Can you work these out from the model? Positions are in its coordinate system, mm. A direction names the side the tool comes from. Round coordinates to 2 decimals unless told otherwise and drop trailing zeros. Loops run counter-clockwise (first coordinate to the right, second up) from the corner with the lowest first, then second, coordinate; pieces in that order, holes last. Notation, with made-up numbers: M 41,-31.5 L 79,-31.5 A7 ccw 79,-23.5 Z; hole C -9.5,-21.5 d8. An arc over 180 degrees is marked long. Return JSON: item names as keys, results as strings.
```python
from build123d import *

# Parameters (mm, degrees)
SKETCH004_R           = 13
SKETCH004_R_2         = 1.6
PAD001_DEPTH          = 3
POLARPATTERN001_COUNT = 3
SKETCH005_R           = 16
SKETCH005_R_2         = 13
PAD002_DEPTH          = 3
CHAMFER003_SIZE       = 0.75


with BuildPart() as part:
    # Sketch004 (on Face1 of Binder001) → Pad001 (new body)
    with BuildSketch(Plane.XZ.offset(-1.75)):
        with BuildLine():
            ThreePointArc((19.050853, 6.088102), (-19.94876, -1.430732), (19.724681, -3.307108))
            Line((24.422075, -4.094689), (19.724681, -3.307108))
            ThreePointArc((24.422075, -4.094689), (31.398835, 2.251935), (23.587776, 7.537972))
            Line((23.587776, 7.537972), (19.050853, 6.088102))
        make_face()
        Circle(SKETCH004_R, mode=Mode.SUBTRACT)
        with Locations((25.414207, 1.822716)):
            Circle(SKETCH004_R_2, mode=Mode.SUBTRACT)
    pad001 = extrude(amount=PAD001_DEPTH)

    # PolarPattern001: Pad001 ×3 about axis
    polarpattern001_axis = Axis((0, 1.75, 0), (0, -1, 0))
    for i in range(1, POLARPATTERN001_COUNT):
        add(pad001.rotate(polarpattern001_axis, i * 360 / POLARPATTERN001_COUNT))

    # Sketch005 (on Face17 of PolarPattern001) → Pad002 (join)
    with BuildSketch(Plane.XZ.offset(1.25)):
        Circle(SKETCH005_R)
        Circle(SKETCH005_R_2, mode=Mode.SUBTRACT)
    extrude(amount=PAD002_DEPTH)

    # Chamfer003
    chamfer003_edges = [part.edges().sort_by_distance(p)[0] for p in [
        (-16, -4.25, 0),
        (31.398835, 1.75, 2.251935),
        (22.073378, 1.75, -3.700898),
        (11.21343, 1.75, -16.560767),
        (-4.759394, 1.75, -21.869587),
        (-13.749184, 1.75, -28.318156),
        (-14.241761, 1.75, -17.265657),
        (-19.94876, 1.75, -1.430732),
        (-16.55992, 1.75, 15.05655),
        (-17.64965, 1.75, 26.066221),
        (-7.831617, 1.75, 20.966555),
        (8.73533, 1.75, 17.991498),
        (21.319315, 1.75, 6.813037),
        (6.5, 1.75, 11.25833),
        (-13, 1.75, 0),
        (6.5, 1.75, -11.25833),
        (23.814207, 1.75, 1.822716),
        (-13.485622, 1.75, 19.71235),
        (-10.328585, 1.75, -21.535066),
    ]]
    chamfer(chamfer003_edges, length=CHAMFER003_SIZE)


solid = part.part
```
Q1. On a 3-axis mill with a long thin cutter (end or side, diameter ignored), from which of +Z, -Z, +X, -X, +Y, -Y can I reach the whole of each face in a straight line? I mean faces 4 (the conical face through (-17.19, 1.62, 25.63)), 5 (the flat face through (-16.06, 1.37, 15.1)), 6 (the flat face through (11.23, -4.25, 6.85)), 7 (the flat face through (22.106, -0.109, -3.706)), 8 (the flat face through (21.351, -0.109, 6.823)). Say none if no direction works.
Results:
{"face 4": "+Y", "face 5": "-X, +Y", "face 6": "+Z, -Z, +X, -X, -Y", "face 7": "-Z, +Y, -Y", "face 8": "+Z, +Y, -Y"}
Q2. Thinking about a two-plate mould opening in X: for faces 1 (the flat face through (-13.69, 1.37, -17.18)), 2 (the flat face through (-7.843, -0.109, 20.998)), 3 (the flat face through (-4, -1.25, 16)), which applies, pulls with the +X half, pulls with the -X half, needs draft (parallel to the pull), parting line crosses it, or undercut?
Results:
{"face 1": "pulls with the -X half", "face 2": "undercut", "face 3": "needs draft"}
Q3. Suppose I cut it at A-A, the plane y = 0. Please give me the cut outline in (x, z).
Results:
{"outline": "M -19.24,-5.47 A20 ccw -12.73,-15.43 L -15.76,-19.1 A6 ccw long -5.27,-24.2 L -4.25,-19.54 A20 ccw 14.36,-13.92 A20 ccw 19.72,-3.31 L 24.42,-4.09 A6 ccw long 23.59,7.54 L 19.05,6.09 A20 ccw 4.88,19.4 A20 ccw -7,18.74 L -8.66,23.2 A6 ccw long -18.32,16.66 L -14.8,13.45 A20 ccw Z; hole C -14.29,21.1 d3.2; hole C 0,0 d26; hole C -11.13,-22.92 d3.2; hole C 25.41,1.82 d3.2"}
Q4. If I drill on line 1 along X through (y, z) = (0.75, 1.5); line 2 along Z through (x, y) = (-15, -0.5); line 3 along Z through (x, y) = (0, -1.1), over which ranges is the centre line in solid material (lowest first)?
Results:
{"line 1": "x = -19.94 to -12.91, 12.91 to 23.85, 26.98 to 31.41", "line 2": "z = -27.5 to -18.18, -13.23 to 13.23, 13.64 to 19.67, 22.53 to 27.06", "line 3": "z = -20 to -13, 13 to 20"}
Q5. I'm going to push flat-ended pins straight in: pin 1 Ø2 at (x, z) = (18, -10) entering from +Y; pin 2 Ø2.5 at (x, z) = (25.41, 1.82) entering from -Y; pin 3 Ø4 at (x, z) = (-14.29, 21.1) entering from -Y; pin 4 Ø1.5 at (y, z) = (-0.5, 8) entering from +X. Where does each tip first touch, or does it pass through?
Results:
{"pin 1": "stops at y = 1.41", "pin 2": "passes through", "pin 3": "stops at y = -1.25", "pin 4": "stops at x = 27.97"}
